from build123d import *

# Parameters (mm, degrees)
SKETCH1_R           = 14
SKETCH1_R_2         = 6
SKETCH1_R_3         = 1.5
BOSS_EXTRUDE1_DEPTH = 10
CHAMFER1_SIZE       = 1
CHAMFER2_SIZE       = 0.5


with BuildPart() as part:
    # Sketch1 → Boss-Extrude1 (new body)
    with BuildSketch(Plane.XY):
        Circle(SKETCH1_R)
        Circle(SKETCH1_R_2, mode=Mode.SUBTRACT)
        with Locations((0, 10.5)):
            Circle(SKETCH1_R_3, mode=Mode.SUBTRACT)
        with Locations((9.09326674, -5.25)):
            Circle(SKETCH1_R_3, mode=Mode.SUBTRACT)
        with Locations((-9.09326674, -5.25)):
            Circle(SKETCH1_R_3, mode=Mode.SUBTRACT)
    extrude(amount=BOSS_EXTRUDE1_DEPTH)

    # Chamfer1
    chamfer1_edges = [part.edges().sort_by_distance(p)[0] for p in [
        (-14, 0, 0),
        (-14, 0, 10),
        (-6, 0, 0),
        (-6, 0, 10),
    ]]
    chamfer(chamfer1_edges, length=CHAMFER1_SIZE)

    # Chamfer2
    chamfer2_edges = [part.edges().sort_by_distance(p)[0] for p in [
        (7.59326674, -5.25, 0),
        (7.59326674, -5.25, 10),
        (-10.59326674, -5.25, 0),
        (-10.59326674, -5.25, 10),
        (-1.5, 10.5, 0),
        (-1.5, 10.5, 10),
    ]]
    chamfer(chamfer2_edges, length=CHAMFER2_SIZE)


solid = part.part
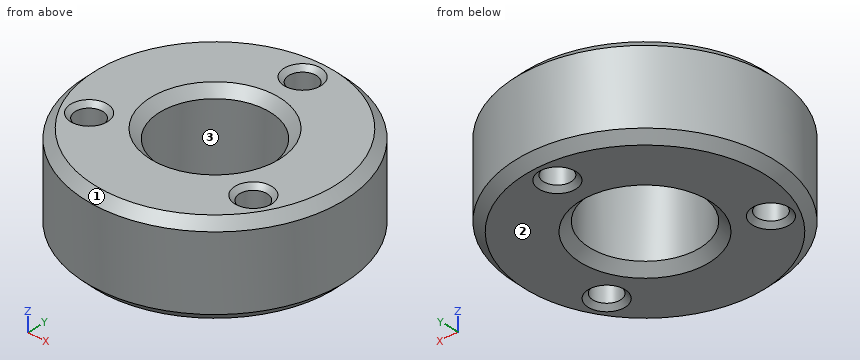
The model under review builds one solid part; all positions refer to its coordinate system, in mm. Face numbers are marked on the shaded views. Round coordinates to 2 decimals unless told otherwise and drop trailing zeros. Loops run counter-clockwise (first coordinate to the right, second up) from the corner with the lowest first, then second, coordinate; pieces in that order, holes last. Notation, with made-up numbers: (-5, 86) -> (25, 86) arc R31 ccw to (25, 115) -> close; hole circle Ø11 at (81.25, 28). An arc over 180 degrees is marked (long way). Answer as CSV lines item,"result".
1) Add section C-C on z = 8.5. Write out the cut boundary in (x, y), plus the area to 3 significant figures.
Geometry results:
outline,"circle Ø28 at (0, 0); hole circle Ø3 at (-9.09, -5.25); hole circle Ø12 at (0, 0); hole circle Ø3 at (0, 10.5); hole circle Ø3 at (9.09, -5.25)"
area,"481 mm²"
2) Add section A-A on y = 0. Write out the cut boundary in (x, z), plus the area to 3 significant figures.
Geometry results:
outline,"(-14, 1) -> (-13, 0) -> (-7, 0) -> (-6, 1) -> (-6, 9) -> (-7, 10) -> (-13, 10) -> (-14, 9) -> close; (6, 1) -> (7, 0) -> (13, 0) -> (14, 1) -> (14, 9) -> (13, 10) -> (7, 10) -> (6, 9) -> close"
area,"156 mm²"
3) For P1, Ø6, axis at x = 1.5, z = 4.5, coming from the +Y side; P2, Ø1.8, axis at x = -9.09, y = -5.25, coming from the -Z side; P3, Ø3, axis at x = -10.5, z = 6, coming from the -Y side; P4, Ø3.5, axis at x = 9.09, y = -5.25, coming from the -Z side, all flat-tipped, find the tip position at first contact; note any pin that passes through.
Geometry results:
P1,"stops at y = 14"
P2,"passes through"
P3,"stops at y = -10.72"
P4,"stops at z = 0.25"
4) To check wall thickness, follow line 1 along Y through (x, z) = (0, 7.5); line 2 along Y through (x, z) = (1.5, 9.75); line 3 along X through (y, z) = (-5.5, 3). State the ranges of each line that lie inside material, in increasing order. Write a range as from..to.
Geometry results:
line 1,"y = -14..-6, 6..9, 12..14"
line 2,"y = -13.16..-6.58, 6.58..9.6, 11.4..13.16"
line 3,"x = -12.87..-10.57, -7.61..-2.4, 2.4..7.61, 10.57..12.87"
5) Draft analysis for pull direction Y (two halves, no side actions). For the marked faces 1, 2 and 3, state which applies: pulls with the +Y half, pulls with the -Y half, needs draft (parallel to the pull), parting line crosses it, or undercut.
Geometry results:
face 1,"parting line crosses it"
face 2,"needs draft"
face 3,"undercut"
6) Add section D-D on y = -5.25. State how many separate pieces and enclosed holes the cut face has, plus the area to 3 significant figures.
Geometry results:
separate pieces,"4"
enclosed holes,"0"
area,"135 mm²"
7) Add section B-B on x = 0. Write out the cut boundary in (y, z).
Geometry results:
outline,"(-14, 1) -> (-13, 0) -> (-7, 0) -> (-6, 1) -> (-6, 9) -> (-7, 10) -> (-13, 10) -> (-14, 9) -> close; (6, 1) -> (7, 0) -> (8.5, 0) -> (9, 0.5) -> (9, 9.5) -> (8.5, 10) -> (7, 10) -> (6, 9) -> close; (12, 0.5) -> (12.5, 0) -> (13, 0) -> (14, 1) -> (14, 9) -> (13, 10) -> (12.5, 10) -> (12, 9.5) -> close"
